Read the model definition and answer for the solid it produces. Units are mm, in the model's axes. A direction names the side the tool comes from. Give positions to 0.01 mm unless a question says otherwise; leave off trailing zeros. Loops run counter-clockwise (first coordinate to the right, second up) from the corner with the lowest first, then second, coordinate; pieces in that order, holes last. Notation, with made-up numbers: (79, 57) - (95, 57) arc R12 ccw to (95, 68) - close; hole circle Ø6 at (-36, 15.5). An arc over 180 degrees is marked (long way). Write each question's results on one line, items separated by ' | '. Start each with the question number.
Q1. Given pin 1 (8 mm diameter, centred on x = 265.5, y = -16.5, fed in from +Z); pin 2 (8 mm diameter, centred on x = 81, z = 30, fed in from -Y); pin 3 (9 mm diameter, centred on x = 430, z = 38.5, fed in from -Y); pin 4 (3 mm diameter, centred on x = 56.5, y = 1, fed in from +Z), each flat-ended and moving along its own axis, determine where each tip first touches the part or whether it passes through.
Q2. Determine the mould class of faces 1 (the flat face through (182.41, -23.875, 8.587)), 2 (the flat face through (291, -11, 57)), 3 (the flat face through (360, -11, 20)) for opening direction Z: +Z half, -Z half, draft (parallel to the pull), parting line (faces both ways), or undercut.
Q3. The part is cut by section A-A, the plane x = 340.5. Write down the section's boundary in (y, z).
Q4. For faces 4 (the flat face through (425, -11, 48.5)), 5 (the flat face through (437, -1, 39)), 6 (the flat face through (182.41, 1.93, 8.83)), 7 (the flat face through (418, -21, 38)), 8 (the cylindrical face through (331.05, -16.71, 38.88)), determine the directions among +Z, -Z, +X, -X, +Y, -Y from which every point of the face is accessible in a straight line to the end or side of a thin tool.
Q5. The part is cut by section C-C, the plane z = 64. Write down the section's boundary in (x, y) (3 decimals), plus the area to 3 significant figures.
Q6. Find the intervals of material crossed by line 1 (Z direction, x = 430, y = -6); line 2 (Y direction, x = 154.5, z = 20); line 3 (X direction, y = -19.5, z = 69.5), in increasing order. Write a range as from..to.
Q7. The part is cut by section B-B, the plane x = 77.5. Write down the section's boundary in (y, z).
Q8. The part is cut by section D-D, the plane x = 387.5. Write down the section's boundary in (y, z), plus the area to 3 significant figures.
```python
from build123d import *

# Parameters (mm, degrees)
SALIENTE_EXTRUIR2_DEPTH = 370
CROQUIS3_R              = 10
CORTAR_EXTRUIR1_DEPTH   = 360
SALIENTE_EXTRUIR3_DEPTH = 40
SALIENTE_EXTRUIR4_DEPTH = 30
CORTAR_EXTRUIR2_REACH   = 449.693
CROQUIS6_R              = 5
CROQUIS7_R              = 19
SALIENTE_EXTRUIR5_DEPTH = 79


with BuildPart() as part:
    # Croquis2 → Saliente-Extruir2 (new body)
    with BuildSketch(Plane(origin=(0, 0, 0), x_dir=(0, 0, -1), z_dir=(1, 0, 0))):
        with BuildLine():
            Line((0, 0), (0, -22))
            Line((0, -22), (-17.417233251, -25.803951615))
            ThreePointArc((-17.417233251, -25.803951615), (-34.834466503, -11), (-17.417233251, 3.803951615))
            Line((-17.417233251, 3.803951615), (0, 0))
        make_face()
    extrude(amount=SALIENTE_EXTRUIR2_DEPTH)

    # Croquis3 → Cortar-Extruir1 (cut)
    with BuildSketch(Plane.ZY):
        with Locations((19.82, -11)):
            Circle(CROQUIS3_R)
    extrude(amount=-CORTAR_EXTRUIR1_DEPTH, mode=Mode.SUBTRACT)

    # Croquis4 → Saliente-Extruir3 (add)
    with BuildSketch(Plane(origin=(370, 0, 0), x_dir=(0, 0, -1), z_dir=(1, 0, 0))):
        with BuildLine():
            Line((0, -11), (0, 2))
            Line((0, 2), (-8.708616626, 9))
            Line((-8.708616626, 9), (-57, 9))
            ThreePointArc((-57, 9), (-77, -11), (-57, -31))
            Line((-57, -31), (-8.708616626, -31))
            Line((-8.708616626, -31), (0, -24))
            Line((0, -24), (0, -11))
        make_face()
    extrude(amount=SALIENTE_EXTRUIR3_DEPTH)

    # Croquis5 → Saliente-Extruir4 (add)
    with BuildSketch(Plane(origin=(410, 0, 0), x_dir=(0, 0, -1), z_dir=(1, 0, 0))):
        with BuildLine():
            Line((-43.5, -1), (-33.5, -1))
            ThreePointArc((-33.5, -1), (-29.964466094, -2.464466094), (-28.5, -6))
            Line((-28.5, -6), (-28.5, -16))
            ThreePointArc((-28.5, -16), (-29.964466094, -19.535533906), (-33.5, -21))
            Line((-33.5, -21), (-43.5, -21))
            ThreePointArc((-43.5, -21), (-47.035533906, -19.535533906), (-48.5, -16))
            Line((-48.5, -16), (-48.5, -6))
            ThreePointArc((-48.5, -6), (-47.035533906, -2.464466094), (-43.5, -1))
        make_face()
    extrude(amount=SALIENTE_EXTRUIR4_DEPTH)

    # Croquis6 → Cortar-Extruir2 (cut, up to next)
    with BuildSketch(Plane(origin=(0, -1, 0), x_dir=(1, 0, 0), z_dir=(0, 1, 0)), mode=Mode.PRIVATE) as cortar_extruir2_sk1:
        with Locations(Location((430, -38.5, 0), (0, 0, 270))):
            Circle(CROQUIS6_R)
    cortar_extruir2_tool1 = extrude(cortar_extruir2_sk1.sketch, amount=-CORTAR_EXTRUIR2_REACH, mode=Mode.PRIVATE) & part.part
    add(cortar_extruir2_tool1.solids().sort_by_distance((430, -1, 38.5))[0], mode=Mode.SUBTRACT)

    # Croquis7 → Saliente-Extruir5 (add)
    with BuildSketch(Plane.ZY.offset(-370)):
        with Locations(Location((57, -11, 0), (0, 0, 180))):
            Circle(CROQUIS7_R)
    extrude(amount=SALIENTE_EXTRUIR5_DEPTH)


solid = part.part
```
Check sheet entries:
1) pin 1: stops at z = 34.76 | pin 2: stops at y = -24.67 | pin 3: passes through | pin 4: stops at z = 30.55
2) face 1: -Z half | face 2: draft | face 3: undercut
3) outline: circle Ø38 at (-11, 57); (-25.8, 17.42) - (-22, 0) - (0, 0) - (3.8, 17.42) arc R15 ccw (long way) to start; hole circle Ø20 at (-11, 19.82)
4) face 4: +Z, +X, +Y, -Y | face 5: +Z, -Z, +X, +Y | face 6: -Z, -X, +Y | face 7: +Z, -Z, +X, -Y | face 8: -X
5) outline: (291, -28.664) - (370, -28.664) - (370, -29.735) - (410, -29.735) - (410, 7.735) - (370, 7.735) - (370, 6.664) - (291, 6.664) - close | area: 4,290 mm^2
6) line 1: z = 28.5..33.5, 43.5..48.5 | line 2: y = -26..-21, -1..4 | line 3: x = 291..410
7) outline: (-25.8, 17.42) - (-22, 0) - (0, 0) - (3.8, 17.42) arc R15 ccw (long way) to start; hole circle Ø20 at (-11, 19.82)
8) outline: (-31, 8.71) - (-24, 0) - (2, 0) - (9, 8.71) - (9, 57) arc R20 ccw to (-31, 57) - close | area: 2,850 mm^2
